Can you work these out from the model? Positions are in its coordinate system, mm. Round coordinates to 2 decimals unless told otherwise and drop trailing zeros. Loops run counter-clockwise (first coordinate to the right, second up) from the corner with the lowest first, then second, coordinate; pieces in that order, holes last. Notation, with made-up numbers: (25, 53.5) -> (57, 53.5) arc R19 ccw to (57, 89.5) -> close; hole circle Ø10 at (24, -3.5). An arc over 180 degrees is marked (long way). Write each question's results on one line, items separated by ' | '.
from build123d import *

# Parameters (mm, degrees)
SKETCH1_R           = 1.75
BOSS_EXTRUDE1_DEPTH = 1.5
FILLET1_R           = 0.5
FILLET2_R           = 0.2
SKETCH5_R           = 1
CUT_EXTRUDE3_DEPTH  = 2.5
FILLET3_R           = 3.1


with BuildPart() as part:
    # Sketch1 → Boss-Extrude1 (new body)
    with BuildSketch(Plane.XY):
        Polygon((0, 0), (0, 6), (39.5, 6), (42, 3.638746799), (39.5, 1.277493599), (11.5, 2.5), (10.489934435, 0), align=None)
        with Locations((39, 3.638746799)):
            Circle(SKETCH1_R, mode=Mode.SUBTRACT)
    extrude(amount=BOSS_EXTRUDE1_DEPTH)

    # Fillet1
    fillet1_edges = [part.edges().sort_by_distance(p)[0] for p in [
        (0, 6, 0.75),
        (11.5, 2.5, 0.75),
        (10.489934435, 0, 0.75),
    ]]
    fillet(fillet1_edges, radius=FILLET1_R)

    # Fillet2
    fillet2_edges = [part.edges().sort_by_distance(p)[0] for p in [
        (39.5, 6, 0.75),
        (42, 3.638746799, 0.75),
        (39.5, 1.277493599, 0.75),
    ]]
    fillet(fillet2_edges, radius=FILLET2_R)

    # Sketch5 → Cut-Extrude3 (cut, through all)
    with BuildSketch(Plane.XY.offset(1.5)):
        with Locations((3.4, 3.2)):
            Circle(SKETCH5_R)
    extrude(amount=-CUT_EXTRUDE3_DEPTH, mode=Mode.SUBTRACT)

    # Fillet3
    fillet3_edges = [part.edges().sort_by_distance(p)[0] for p in [
        (0, 0, 0.75),
    ]]
    fillet(fillet3_edges, radius=FILLET3_R)


solid = part.part
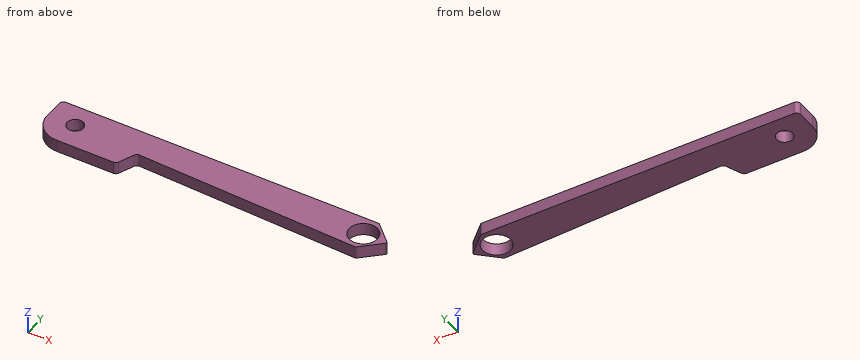
1. If we section it at B-B (z = 0.9): List the corners of the cut face in (x, y) for me.
Final values:
outline: (0, 3.1) arc R3.1 ccw to (3.1, 0) -> (10.15, 0) arc R0.5 ccw to (10.62, 0.31) -> (11.37, 2.17) arc R0.5 cw to (11.85, 2.48) -> (39.42, 1.28) arc R0.2 ccw to (39.56, 1.34) -> (41.85, 3.49) arc R0.2 ccw to (41.85, 3.78) -> (39.56, 5.95) arc R0.2 ccw to (39.42, 6) -> (0.5, 6) arc R0.5 ccw to (0, 5.5) -> close; hole circle Ø2 at (3.4, 3.2); hole circle Ø3.5 at (39, 3.64)
2. If we section it at D-D (x = 18.5): List the corners of the cut face in (y, z) for me, then the cut area to 3 significant figures.
Final values:
outline: (2.19, 0) -> (6, 0) -> (6, 1.5) -> (2.19, 1.5) -> close | area: 5.71 mm2
3. Please list where these lines run through material, in increasing order: line 1 (Y direction, x = 3.4, z = 0.9); line 2 (X direction, y = 5, z = 0.8); line 3 (X direction, y = 5.1, z = 1). Write a range as from..to.
Final values:
line 1: 0..2.2, 4.2..6 | line 2: 0..37.9, 40.1..40.56 | line 3: 0..38.04, 39.96..40.45
4. If we section it at C-C (x = 31.5): List the corners of the cut face in (y, z) for me, then the cut area to 3 significant figures.
Final values:
outline: (1.63, 0) -> (6, 0) -> (6, 1.5) -> (1.63, 1.5) -> close | area: 6.56 mm2
5. If we section it at A-A (x = 39): List the corners of the cut face in (y, z) for me, then the cut area to 3 significant figures.
Final values:
outline: (1.3, 0) -> (1.89, 0) -> (1.89, 1.5) -> (1.3, 1.5) -> close; (5.39, 0) -> (6, 0) -> (6, 1.5) -> (5.39, 1.5) -> close | area: 1.80 mm2
